Geometry check sheet. Reference: the model listing, model coordinates, mm. A direction names the side the tool comes from. Give positions to 0.01 mm unless a question says otherwise; leave off trailing zeros. Write each loop counter-clockwise with the first axis right and the second up, starting at its lowest first coordinate (ties: lowest second). Pieces come first, ordered by that corner, then holes. Notation, with made-up numbers: (69, 35) -> (94, 35) arc R26 cw to (94, 74) -> close; hole circle Ø11 at (43.5, 44). An arc over 180 degrees is marked (long way). Write item = value, one per line. Start each with the question number.
1. Set-up check for faces 1 (the flat face through (-5.742, 1.451, -3.254)), 2 (the cylindrical face through (0.09, 9.54, -11.6)), 3 (the cylindrical face through (-7.622, 4.902, 3.832)): record each of +Z, -Z, +X, -X, +Y, -Y from which the full face is reachable in a straight line by a thin tool's end or side.
2. Depth check by flat-ended pin: P1, Ø1.3, axis at x = -9, z = 0, coming from the +Y side; P2, Ø9.5, axis at x = 0, z = 0, coming from the -Y side; P3, Ø4, axis at x = -4, y = 5, coming from the -Z side; P4, Ø2, axis at x = -10, y = 9, coming from the -Z side. Enter the tip coordinate at first touch or a pass-through.
3. Thickness scan on line 1 along X through (y, z) = (8.5, 0); line 2 along X through (y, z) = (3.5, 0); line 3 along Z through (x, y) = (-8.5, 1.25). Record the ranges inside material, lowest first.
4. Cross-section at C-C, the plane z = 18.5. Record the cut outline in (x, y), plus the area to 3 significant figures.
5. Cross-section at A-A, the plane x = 0. State how many separate pieces and enclosed holes the cut face has, plus the area to 3 significant figures.
```python
from build123d import *
from build123d.topology import SkipClean

# Parameters (mm, degrees)
SKETCH_1_R          = 15.75
SKETCH_1_R_2        = 5.25
EXTRUDE_1_DEPTH     = 12
EXTRUDE_START       = 2
SKETCH_2_R          = 5.25
EXTRUDE_2_DEPTH     = 2
CUT_EXTRUDE_1_DEPTH = 7
SKETCH_5_R          = 1.1
CUT_EXTRUDE_2_DEPTH = 38.348432031
SKETCH_6_R          = 2.1
CUT_EXTRUDE_3_DEPTH = 5
CHAMFER_1_SIZE      = 1
CUT_EXTRUDE_4_DEPTH = 38.348432031
FILLET_1_R          = 2


with BuildPart() as part:
    # Эскиз1 → Бобышка-Вытянуть1 (new body)
    with BuildSketch(Plane(origin=(0, 0, 0), x_dir=(1, 0, 0), z_dir=(0, 1, 0))):
        with Locations(Location((0, 0, 0), (0, 0, 270))):
            Circle(SKETCH_1_R)
        with Locations(Location((0, 0, 0), (0, 0, 270))):
            Circle(SKETCH_1_R_2, mode=Mode.SUBTRACT)
    extrude(amount=EXTRUDE_1_DEPTH)

    # Эскиз2 → Бобышка-Вытянуть2 (add)
    with SkipClean():  # the faces are left unmerged after this step: merging them gives an invalid solid
        with BuildSketch(Plane.XZ.offset(EXTRUDE_START)):
            with BuildLine():
                Line((-8.660254038, 20.5), (-22.083647797, -2.75))
                ThreePointArc((-22.083647797, -2.75), (-22.083647797, -12.75), (-13.423393759, -17.75))
                Line((-13.423393759, -17.75), (13.423393759, -17.75))
                ThreePointArc((13.423393759, -17.75), (22.083647797, -12.75), (22.083647797, -2.75))
                Line((22.083647797, -2.75), (8.660254038, 20.5))
                ThreePointArc((8.660254038, 20.5), (0, 25.5), (-8.660254038, 20.5))
            make_face()
            with Locations(Location((0, 0, 0), (0, 0, 270))):
                Circle(SKETCH_2_R, mode=Mode.SUBTRACT)
        extrude(amount=-EXTRUDE_2_DEPTH)

    # Эскиз3 → Вырез-Вытянуть1 (cut)
    with BuildSketch(Plane.XZ.offset(2)):
        Polygon((3.810511777, 6.6), (-3.810511777, 6.6), (-7.621023553, 0), (-3.810511777, -6.6), (3.810511777, -6.6), (7.621023553, 0), align=None)
    extrude(amount=-CUT_EXTRUDE_1_DEPTH, mode=Mode.SUBTRACT)

    # Эскиз5 → Вырез-Вытянуть2 (cut, through all)
    with BuildSketch(Plane(origin=(0, 12, 0), x_dir=(1, 0, 0), z_dir=(0, 1, 0))):
        with Locations(Location((0, 9.5, 0), (0, 0, 270))):
            Circle(SKETCH_5_R)
        with Locations(Location((9.5, 0, 0), (0, 0, 270))):
            Circle(SKETCH_5_R)
        with Locations(Location((0, -9.5, 0), (0, 0, 270))):
            Circle(SKETCH_5_R)
        with Locations(Location((-9.5, 0, 0), (0, 0, 270))):
            Circle(SKETCH_5_R)
    extrude(amount=-CUT_EXTRUDE_2_DEPTH, mode=Mode.SUBTRACT)

    # Эскиз6 → Вырез-Вытянуть3 (cut)
    with BuildSketch(Plane(origin=(0, 12, 0), x_dir=(1, 0, 0), z_dir=(0, 1, 0))):
        with Locations(Location((0, 9.5, 0), (0, 0, 270))):
            Circle(SKETCH_6_R)
        with Locations(Location((9.5, 0, 0), (0, 0, 270))):
            Circle(SKETCH_6_R)
        with Locations(Location((0, -9.5, 0), (0, 0, 270))):
            Circle(SKETCH_6_R)
        with Locations(Location((-9.5, 0, 0), (0, 0, 270))):
            Circle(SKETCH_6_R)
    extrude(amount=-CUT_EXTRUDE_3_DEPTH, mode=Mode.SUBTRACT)

    # Фаска1
    chamfer_1_edges = [part.edges().sort_by_distance(p)[0] for p in [
        (0, 12, -15.75),
        (0, 12, -5.25),
    ]]
    chamfer(chamfer_1_edges, length=CHAMFER_1_SIZE)

    # Эскиз7 → Вырез-Вытянуть4 (cut, through all)
    with BuildSketch(Plane(origin=(0, 12, 0), x_dir=(1, 0, 0), z_dir=(0, 1, 0))):
        with BuildLine():
            Line((5.2, 11.914696807), (3.2, 7.332121112))
            ThreePointArc((3.2, 7.332121112), (5.656854249, 5.656854249), (7.332121112, 3.2))
            Line((7.332121112, 3.2), (11.914696807, 5.2))
            ThreePointArc((11.914696807, 5.2), (9.192388155, 9.192388155), (5.2, 11.914696807))
        make_face()
        with BuildLine():
            Line((11.914696807, -5.2), (7.332121112, -3.2))
            ThreePointArc((7.332121112, -3.2), (5.656854249, -5.656854249), (3.2, -7.332121112))
            Line((3.2, -7.332121112), (5.2, -11.914696807))
            ThreePointArc((5.2, -11.914696807), (9.192388155, -9.192388155), (11.914696807, -5.2))
        make_face()
        with BuildLine():
            Line((-5.2, -11.914696807), (-3.2, -7.332121112))
            ThreePointArc((-3.2, -7.332121112), (-5.656854249, -5.656854249), (-7.332121112, -3.2))
            Line((-7.332121112, -3.2), (-11.914696807, -5.2))
            ThreePointArc((-11.914696807, -5.2), (-9.192388155, -9.192388155), (-5.2, -11.914696807))
        make_face()
        with BuildLine():
            Line((-11.914696807, 5.2), (-7.332121112, 3.2))
            ThreePointArc((-7.332121112, 3.2), (-5.656854249, 5.656854249), (-3.2, 7.332121112))
            Line((-3.2, 7.332121112), (-5.2, 11.914696807))
            ThreePointArc((-5.2, 11.914696807), (-9.192388155, 9.192388155), (-11.914696807, 5.2))
        make_face()
    extrude(amount=-CUT_EXTRUDE_4_DEPTH, mode=Mode.SUBTRACT)

    # Скругление1
    fillet_1_edges = [part.edges().sort_by_distance(p)[0] for p in [
        (-5.2, 5, -11.914696807),
        (-3.2, 5, -7.332121112),
        (-7.332121112, 5, -3.2),
        (-11.914696807, 5, -5.2),
        (-11.914696807, 5, 5.2),
        (-7.332121112, 5, 3.2),
        (-3.2, 5, 7.332121112),
        (-5.2, 5, 11.914696807),
        (5.2, 5, 11.914696807),
        (3.2, 5, 7.332121112),
        (7.332121112, 5, 3.2),
        (11.914696807, 5, 5.2),
        (11.914696807, 5, -5.2),
        (7.332121112, 5, -3.2),
        (3.2, 5, -7.332121112),
        (5.2, 5, -11.914696807),
    ]]
    fillet(fillet_1_edges, radius=FILLET_1_R)


solid = part.part
```
Answers:
q1.face_1 = -Y
q1.face_2 = +Y
q1.face_3 = +Y, -Y
q2.P1 = 7
q2.P2 = through
q2.P3 = -15.62
q2.P4 = -12.93
q3.line_1 = -15.75 to -11.6, -7.4 to -5.25, 5.25 to 7.4, 11.6 to 15.75
q3.line_2 = -15.75 to -10.6, -8.4 to -7.62, 7.62 to 8.4, 10.6 to 15.75
q3.line_3 = -13.26 to -9.84, -3.78 to -0.46, 0.46 to 3.78, 9.84 to 13.26
q4.outline = (-9.81, -2) -> (9.81, -2) -> (9.81, 0) -> (-9.81, 0) -> close
q4.area = 39.3 mm^2
q5.separate_pieces = 4
q5.enclosed_holes = 0
q5.area = 215 mm^2
